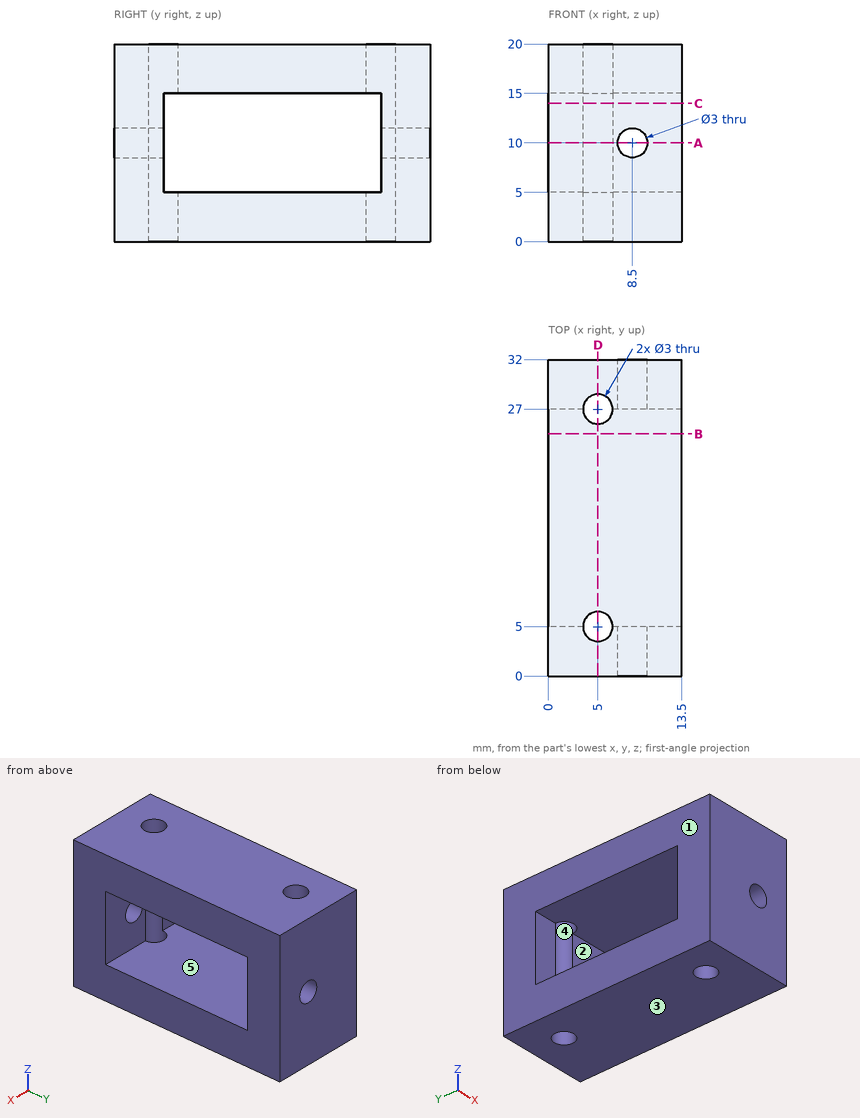
Verification items for this drawing (mm, ordinates from the low corner). A direction names the side the tool comes from. Give positions to 0.01 mm unless a question says otherwise; leave off trailing zeros. Loops run counter-clockwise (first coordinate to the right, second up) from the corner with the lowest first, then second, coordinate; pieces in that order, holes last. Notation, with made-up numbers: M -22,74 L -7,74 A21 cw -7,85 Z; hole C 14,66 d8. An arc over 180 degrees is marked long. Answer as CSV lines item,"result".
Item 1: Cross-section at C-C on z = 14. Record the cut outline in (x, y).
Values:
outline,"M 0,0 L 13.5,0 L 13.5,5 L 6.5,5 A1.5 cw 3.5,5 L 0,5 Z; M 0,27 L 3.5,27 A1.5 cw 6.5,27 L 13.5,27 L 13.5,32 L 0,32 Z"
Item 2: Release check for a two-part mould opening along Z. For the marked faces 1, 2 and 3 record: pulls with the +Z half, pulls with the -Z half, needs draft (parallel to the pull), parting line crosses it, or undercut.
Values:
face 1,"needs draft"
face 2,"undercut"
face 3,"pulls with the -Z half"
Item 3: Cross-section at A-A on z = 10. Record the cut outline in (x, y), and give its area (3 significant figures).
Values:
outline,"M 0,0 L 7,0 L 7,5 L 6.5,5 A1.5 cw 3.5,5 L 0,5 Z; M 0,27 L 3.5,27 A1.5 cw 6.5,27 L 7,27 L 7,32 L 0,32 Z; M 10,0 L 13.5,0 L 13.5,5 L 10,5 Z; M 10,27 L 13.5,27 L 13.5,32 L 10,32 Z"
area,"97.9 mm²"
Item 4: Material ranges on line 1 (Y direction, x = 5, z = 15.5); line 2 (Z direction, x = 2.25, y = 11); line 3 (Y direction, x = 5, z = 14.5), recorded low to high.
Values:
line 1,"y = 0 to 3.5, 6.5 to 25.5, 28.5 to 32"
line 2,"z = 0 to 5, 15 to 20"
line 3,"y = 0 to 3.5, 28.5 to 32"
Item 5: Depth check by flat-ended pin: P1, Ø5.5, axis at x = 10, z = 9, coming from the -Y side. Enter the tip coordinate at first touch or a pass-through.
Values:
P1,"stops at y = 0"
Item 6: Cross-section at B-B on y = 24.5. Record the cut outline in (x, z).
Values:
outline,"M 0,0 L 13.5,0 L 13.5,5 L 0,5 Z; M 0,15 L 13.5,15 L 13.5,20 L 0,20 Z"
Item 7: Access from +Z, -Z, +X, -X, +Y, -Y to the whole of each face (thin tool, end or side, straight path). Record for the marked faces 4 and 5.
Values:
face 4,"+Z, -Z"
face 5,"+X, -X"
Item 8: Cross-section at D-D on x = 5. Record the cut outline in (y, z).
Values:
outline,"M 0,0 L 3.5,0 L 3.5,20 L 0,20 Z; M 6.5,0 L 25.5,0 L 25.5,5 L 6.5,5 Z; M 6.5,15 L 25.5,15 L 25.5,20 L 6.5,20 Z; M 28.5,0 L 32,0 L 32,20 L 28.5,20 Z"
